```python
from build123d import *

# Parameters (mm, degrees)
F0_W     = 150.06873
F0_H     = 83.760024
F1_DEPTH = 63.5
F3_D     = 38.1
F5_D     = 38.1


with BuildPart() as f1:
    # F0 (on Front) → F1 (new body)
    with BuildSketch(Plane.XZ):
        Rectangle(F0_W, F0_H)
    extrude(amount=F1_DEPTH)

    # F3 (through all)
    with Locations(Plane(origin=(0, 0, 0), x_dir=(-1, 0, 0), z_dir=(0, 1, 0))):
        with Locations((-39.070934, 0)):
            Hole(F3_D / 2)

    # F5 (through all)
    with Locations(Plane(origin=(0, 0, 0), x_dir=(-1, 0, 0), z_dir=(0, 1, 0))):
        with Locations((40.15404, 0)):
            Hole(F5_D / 2)


solid = f1.part
```
The listing builds one solid part. Answer for the finished solid, in the listing's coordinates (mm). Give positions to 0.01 mm unless a question says otherwise; leave off trailing zeros. Order: outer loops, then holes, each group sorted by start corner. A loop starts at its lowest first (then second) coordinate and runs counter-clockwise, first axis right, second up. Notation, with made-up numbers: (18, 35) -> (42, 35) arc R4 cw to (42, 39) -> close; hole circle Ø3 at (66, -33). An arc over 180 degrees is marked (long way). Answer as a JSON object with one key per item and string values. Group by question number.
Item 1: The part is cut by section C-C on y = -27. Write down the section's boundary in (x, z).
Item 2: The part is cut by section B-B on x = -38. Write down the section's boundary in (y, z), and give its area (3 significant figures).
Item 3: The part is cut by section A-A on z = 0. Write down the section's boundary in (x, y), and give its area (3 significant figures).
Item 4: Consider L1, parallel to X at y = -8, z = -1; L2, parallel to X at y = -10.5, z = -10.5; L3, parallel to Z at x = 39, y = -30. Determine where each line is inside the solid, lowest interval first. Write a range as from..to.
Item 5: The part is cut by section D-D on z = -9.5. Write down the section's boundary in (x, y).
Item 6: Determine the mould class of faces 1 (the cylindrical face through (20.04, -32.19, 0.84)), 2 (the flat face through (75.034, -31, -1)), 3 (the flat face through (-1, 0, 1)) for opening direction X: pulls with the +X half, pulls with the -X half, needs draft (parallel to the pull), parting line crosses it, or undercut.
Result set:
{
 "1": {"outline": "(-75.03, -41.88) -> (75.03, -41.88) -> (75.03, 41.88) -> (-75.03, 41.88) -> close; hole circle Ø38.1 at (-40.15, 0); hole circle Ø38.1 at (39.07, 0)"},
 "2": {"outline": "(-63.5, -41.88) -> (0, -41.88) -> (0, -18.93) -> (-63.5, -18.93) -> close; (-63.5, 18.93) -> (0, 18.93) -> (0, 41.88) -> (-63.5, 41.88) -> close", "area": "2,910 mm²"},
 "3": {"outline": "(-75.03, -63.5) -> (-59.2, -63.5) -> (-59.2, 0) -> (-75.03, 0) -> close; (-21.1, -63.5) -> (20.02, -63.5) -> (20.02, 0) -> (-21.1, 0) -> close; (58.12, -63.5) -> (75.03, -63.5) -> (75.03, 0) -> (58.12, 0) -> close", "area": "4,690 mm²"},
 "4": {"L1": "-75.03..-59.18, -21.13..20.05, 58.09..75.03", "L2": "-75.03..-56.05, -24.26..23.18, 54.97..75.03", "L3": "-41.88..-19.05, 19.05..41.88"},
 "5": {"outline": "(-75.03, -63.5) -> (-56.67, -63.5) -> (-56.67, 0) -> (-75.03, 0) -> close; (-23.64, -63.5) -> (22.56, -63.5) -> (22.56, 0) -> (-23.64, 0) -> close; (55.58, -63.5) -> (75.03, -63.5) -> (75.03, 0) -> (55.58, 0) -> close"},
 "6": {"face 1": "undercut", "face 2": "pulls with the +X half", "face 3": "needs draft"}
}
